Geometry: final body of the model. Coordinates: model frame, mm. A direction names the side the tool comes from. Give positions to 0.01 mm unless a question says otherwise; leave off trailing zeros. Write each loop counter-clockwise with the first axis right and the second up, starting at its lowest first coordinate (ties: lowest second). Pieces come first, ordered by that corner, then holes. Notation, with made-up numbers: (14.25, -18) -> (24.25, -18) arc R15 ccw to (24.25, -10) -> close; hole circle Ø8 at (20, 77). An arc over 180 degrees is marked (long way). Answer in a Markdown table with one row per item. Add a question column.
Item 1: Access query for faces 1 (the flat face through (35, 3, -48)), 2 (the flat face through (35, 0, -48)). Directions: +Z, -Z, +X, -X, +Y, -Y. A direction counts if a zero-diameter tool reaches every point of the face in a straight line with its end or side. Return the directions, or none.
Item 2: Material intervals for probe 1 along Z at (x, y) = (43.25, 3.25); probe 2 along Y at (x, z) = (33.5, -52.25); probe 3 along Y at (x, z) = (33.25, -46), sorted ascending. Write a range as from..to.
Item 3: First-contact query: P1, Ø3, axis at x = 40.5, z = -47, coming from the +Y side; P2, Ø1.9, axis at x = 30.34, z = -47.72, coming from the +Y side; P3, Ø5, axis at x = 38.5, z = -50.5, coming from the +Y side. Flat tips, straight axial feed; report the tip coordinate or a pass-through.
Item 4: Section query D-D on z = -48. Output: boundary loops of the cut face in (x, y), plus the area to 3 significant figures.
Item 5: Section query A-A on z = -52.75. Output: boundary loops of the cut face in (x, y).
Item 6: Section query C-C on x = 40.75. Output: boundary loops of the cut face in (y, z).
Item 7: Section query B-B on y = 4.5. Output: boundary loops of the cut face in (x, z), plus the area to 3 significant figures.
Item 8: Draft query along Z for faces 3 (the flat face through (35, 9, -44.219)), 4 (the flat face through (42.286, 8.983, -42.74)), 5 (the flat face through (35, 7, -41.219)). Return one class per face: +Z half, -Z half, draft (parallel to the pull), parting line (faces both ways), or undercut.
```python
from build123d import *

# Parameters (mm, degrees)
SKETCH_1_W                  = 20
SKETCH_1_H                  = 7
EXTRUDE_1_DEPTH             = 3
EXTRUDE_2_DEPTH             = 3
EXTRUDE_3_DEPTH             = 3
HOLE_WIZARD_3_2_3_2_1_D     = 3.2
HOLE_WIZARD_3_2_3_2_1_DEPTH = 17.544769413
HOLE_WIZARD_5_0_5_1_D       = 5
HOLE_WIZARD_5_0_5_1_DEPTH   = 3
HOLE_WIZARD_5_0_5_2_D       = 5


with BuildPart() as part:
    # 草图1 → 凸台-拉伸1 (new body)
    with BuildSketch(Plane(origin=(0, 3, 0), x_dir=(1, 0, 0), z_dir=(0, 1, 0))):
        with Locations((35.343075637, 47.719425868)):
            Rectangle(SKETCH_1_W, SKETCH_1_H)
    extrude(amount=-EXTRUDE_1_DEPTH)

    # 草图2 → 凸台-拉伸2 (add)
    with BuildSketch(Plane.XY.offset(-44.219425868)):
        with BuildLine():
            Line((45.343075637, 0), (25.343075637, 0))
            Line((25.343075637, 0), (25.343075637, 3))
            Line((25.343075637, 3), (31.372178722, 14.8))
            ThreePointArc((31.372178722, 14.8), (35.343075637, 17.544764106), (39.313972553, 14.8))
            Line((39.313972553, 14.8), (45.343075637, 3))
            Line((45.343075637, 3), (45.343075637, 0))
        make_face()
    extrude(amount=EXTRUDE_2_DEPTH)

    # 草图3 → 凸台-拉伸3 (add)
    with BuildSketch(Plane(origin=(0, 0, -51.219425868), x_dir=(-1, 0, 0), z_dir=(0, 0, -1))):
        with BuildLine():
            Line((-25.343075637, 0), (-45.343075637, 0))
            Line((-45.343075637, 0), (-45.343075637, 3))
            Line((-45.343075637, 3), (-39.313966075, 14.800005308))
            ThreePointArc((-39.313966075, 14.800005308), (-35.34306916, 17.544769413), (-31.372172244, 14.800005308))
            Line((-31.372172244, 14.800005308), (-25.343075637, 3))
            Line((-25.343075637, 3), (-25.343075637, 0))
        make_face()
    extrude(amount=EXTRUDE_3_DEPTH)

    # Ø3.2 (3.2) 直径孔1
    with Locations(Plane(origin=(0, 0, 0), x_dir=(-1, 0, 0), z_dir=(0, -1, 0))):
        with Locations((-40.343075637, 47.719425868), (-30.343075637, 47.719425868)):
            Hole(HOLE_WIZARD_3_2_3_2_1_D / 2, depth=HOLE_WIZARD_3_2_3_2_1_DEPTH)

    # Ø5.0 (5) 直径孔1
    with Locations(Plane(origin=(0, 0, -54.219425868), x_dir=(-1, 0, 0), z_dir=(0, 0, -1))):
        with Locations((-35.34306916, 13.300005308)):
            Hole(HOLE_WIZARD_5_0_5_1_D / 2, depth=HOLE_WIZARD_5_0_5_1_DEPTH)

    # Ø5.0 (5) 直径孔2 (through all)
    with Locations(Plane(origin=(0, 0, -44.219425868), x_dir=(-1, 0, 0), z_dir=(0, 0, -1))):
        with Locations((-35.34306916, 13.300005308)):
            Hole(HOLE_WIZARD_5_0_5_2_D / 2)


solid = part.part
```
Findings below:
| question | item | result |
|---|---|---|
| 1 | face 1 | +X, -X, +Y |
| 1 | face 2 | +Z, -Z, +X, -X, -Y |
| 2 | probe 1 | z = -54.22..-51.22, -44.22..-41.22 |
| 2 | probe 2 | y = 0..11.61, 14.99..17.12 |
| 2 | probe 3 | y = 0..3 |
| 3 | P1 | stops at y = 3 |
| 3 | P2 | passes through |
| 3 | P3 | stops at y = 17.48 |
| 4 | outline | (25.34, 0) -> (28.77, 0) -> (28.77, 3) -> (25.34, 3) -> close; (31.92, 0) -> (38.77, 0) -> (38.77, 3) -> (31.92, 3) -> close; (41.92, 0) -> (45.34, 0) -> (45.34, 3) -> (41.92, 3) -> close |
| 4 | area | 41.1 mm^2 |
| 5 | outline | (25.34, 0) -> (45.34, 0) -> (45.34, 3) -> (39.31, 14.8) arc R4.24 ccw to (31.37, 14.8) -> (25.34, 3) -> close; hole circle Ø5 at (35.34, 13.3) |
| 6 | outline | (0, -54.22) -> (11.99, -54.22) -> (11.99, -51.22) -> (3, -51.22) -> (3, -49.27) -> (0, -49.27) -> close; (0, -46.17) -> (3, -46.17) -> (3, -44.22) -> (11.99, -44.22) -> (11.99, -41.22) -> (0, -41.22) -> close |
| 7 | outline | (26.11, -54.22) -> (44.58, -54.22) -> (44.58, -51.22) -> (26.11, -51.22) -> close; (26.11, -44.22) -> (44.58, -44.22) -> (44.58, -41.22) -> (26.11, -41.22) -> close |
| 7 | area | 111 mm^2 |
| 8 | face 3 | undercut |
| 8 | face 4 | draft |
| 8 | face 5 | +Z half |
